Source: CAD feature listing. Evaluate the final solid. Frame: model axes, mm. A direction names the side the tool comes from. Give positions to 0.01 mm unless a question says otherwise; leave off trailing zeros. Write each loop counter-clockwise with the first axis right and the second up, starting at its lowest first coordinate (ties: lowest second). Pieces come first, ordered by that corner, then holes. Notation, with made-up numbers: (-36.75, 55) -> (-18.75, 55) arc R8 ccw to (-18.75, 67) -> close; hole circle Ø4 at (6, -8.5). An arc over 180 degrees is marked (long way). Answer as a JSON object with one key per item and string values. Group by question number.
Item 1: Access query for faces 4 (the face through (81, 8, -26)), 5 (the face through (191, 4, -71.204)). Directions: +Z, -Z, +X, -X, +Y, -Y. A direction counts if a zero-diameter tool reaches every point of the face in a straight line with its end or side. Return the directions, or none.
Item 2: First-contact query: pin 1 Ø3 at (x, z) = (79.79, -50.39) entering from +Y. Flat tip, straight axial feed; report the tip coordinate or a pass-through.
Item 3: Pull-direction query (Z, two-part tool) for faces 1 (the face through (81, 4, 35.296)), 2 (the face through (191, 4, -68.204)), 3 (the face through (81, 4, -84.704)); classes: pulls with the +Z half, pulls with the -Z half, needs draft (parallel to the pull), parting line crosses it, or undercut.
Item 4: Ray query, probe 1 along X at (y, z) = (7.5, -41); probe 2 along Z at (x, y) = (195.5, 0.5); probe 3 along Z at (x, y) = (213.5, 2.25). Return the intervals inside material, ascending. Write a range as from..to.
Item 5: Section query A-A on z = -19. Return the cut outline in (x, y), plus the area to 3 significant figures.
Item 6: Section query B-B on y = 6.75. Give the number of separate pieces and of enclosed holes in the cut face, plus the area to 3 significant figures.
from build123d import *

# Parameters (mm, degrees)
SKETCH1_W           = 300
SKETCH1_H           = 120
BOSS_EXTRUDE1_DEPTH = 8
SKETCH2_R           = 1.636
SKETCH2_R_2         = 1.687
CUT_EXTRUDE1_DEPTH  = 8
CUT_EXTRUDE2_DEPTH  = 8
CUT_EXTRUDE3_DEPTH  = 8
SKETCH2_5_R         = 1.636
CUT_EXTRUDE4_DEPTH  = 8
SKETCH5_R           = 2
CUT_EXTRUDE5_DEPTH  = 8
SKETCH5_3_R         = 2
CUT_EXTRUDE6_DEPTH  = 8
CUT_EXTRUDE7_DEPTH  = 8
SKETCH9_R           = 1.5
CUT_EXTRUDE9_DEPTH  = 10
SKETCH8_R           = 1.5
CUT_EXTRUDE10_DEPTH = 10
SKETCH10_R          = 1.687
SKETCH10_R_2        = 1.636
CUT_EXTRUDE11_DEPTH = 10
SKETCH10_3_R        = 2
CUT_EXTRUDE12_DEPTH = 10
SKETCH10_4_R        = 2
CUT_EXTRUDE13_DEPTH = 10


with BuildPart() as part:
    # Sketch1 → Boss-Extrude1 (new body)
    with BuildSketch(Plane(origin=(0, 0, 0), x_dir=(1, 0, 0), z_dir=(0, 1, 0))):
        with Locations((83.012516048, 24.703699284)):
            Rectangle(SKETCH1_W, SKETCH1_H)
    extrude(amount=BOSS_EXTRUDE1_DEPTH)

    # Sketch2 → Cut-Extrude1 (cut)
    with BuildSketch(Plane(origin=(0, 8, 0), x_dir=(1, 0, 0), z_dir=(0, 1, 0))):
        with Locations((79.785470733, 50.392260228)):
            Circle(SKETCH2_R)
        with Locations((74.502270733, 49.630260228)):
            Circle(SKETCH2_R_2)
        with Locations((81.055470733, 2.132260228)):
            Circle(SKETCH2_R)
        with Locations((155.985470733, 2.132260228)):
            Circle(SKETCH2_R)
    extrude(amount=-CUT_EXTRUDE1_DEPTH, mode=Mode.SUBTRACT)

    # Sketch2<3> → Cut-Extrude2 (cut)
    with BuildSketch(Plane(origin=(0, 8, 0), x_dir=(1, 0, 0), z_dir=(0, 1, 0))):
        with BuildLine():
            Line((-58.487483952, -8.046300716), (-58.487483952, 57.453699284))
            ThreePointArc((-58.487483952, 57.453699284), (-56.987483952, 58.953699284), (-55.487483952, 57.453699284))
            Line((-55.487483952, 57.453699284), (-55.487483952, -8.046300716))
            ThreePointArc((-55.487483952, -8.046300716), (-56.987483952, -9.546300716), (-58.487483952, -8.046300716))
        make_face()
    extrude(amount=-CUT_EXTRUDE2_DEPTH, mode=Mode.SUBTRACT)

    # Sketch2<4> → Cut-Extrude3 (cut)
    with BuildSketch(Plane(origin=(0, 8, 0), x_dir=(1, 0, 0), z_dir=(0, 1, 0))):
        with BuildLine():
            Line((126.512516048, -8.046300716), (126.512516048, 57.453699284))
            ThreePointArc((126.512516048, 57.453699284), (128.012516048, 58.953699284), (129.512516048, 57.453699284))
            Line((129.512516048, 57.453699284), (129.512516048, -8.046300716))
            ThreePointArc((129.512516048, -8.046300716), (128.012516048, -9.546300716), (126.512516048, -8.046300716))
        make_face()
    extrude(amount=-CUT_EXTRUDE3_DEPTH, mode=Mode.SUBTRACT)

    # Sketch2<5> → Cut-Extrude4 (cut)
    with BuildSketch(Plane(origin=(0, 8, 0), x_dir=(1, 0, 0), z_dir=(0, 1, 0))):
        with Locations((162.335470733, 50.392260228)):
            Circle(SKETCH2_5_R)
    extrude(amount=-CUT_EXTRUDE4_DEPTH, mode=Mode.SUBTRACT)

    # Sketch5 → Cut-Extrude5 (cut)
    with BuildSketch(Plane(origin=(0, 8, 0), x_dir=(1, 0, 0), z_dir=(0, 1, 0))):
        with Locations((83.012516048, -20.296300716)):
            Circle(SKETCH5_R)
    extrude(amount=-CUT_EXTRUDE5_DEPTH, mode=Mode.SUBTRACT)

    # Sketch5<3> → Cut-Extrude6 (cut)
    with BuildSketch(Plane(origin=(0, 8, 0), x_dir=(1, 0, 0), z_dir=(0, 1, 0))):
        with Locations((83.012516048, 69.703699284)):
            Circle(SKETCH5_3_R)
    extrude(amount=-CUT_EXTRUDE6_DEPTH, mode=Mode.SUBTRACT)

    # Sketch6 → Cut-Extrude7 (cut)
    with BuildSketch(Plane(origin=(0, 8, 0), x_dir=(1, 0, 0), z_dir=(0, 1, 0))):
        with BuildLine():
            Line((180.768543767, 71.203699284), (201.803443745, 71.203699284))
            ThreePointArc((201.803443745, 71.203699284), (203.303443745, 69.703699284), (201.803443745, 68.203699284))
            Line((201.803443745, 68.203699284), (180.768543767, 68.203699284))
            ThreePointArc((180.768543767, 68.203699284), (179.268543767, 69.703699284), (180.768543767, 71.203699284))
        make_face()
        with BuildLine():
            Line((180.768543767, -18.796300716), (200.303443745, -18.796300716))
            ThreePointArc((200.303443745, -18.796300716), (201.803443745, -20.296300716), (200.303443745, -21.796300716))
            Line((200.303443745, -21.796300716), (180.768543767, -21.796300716))
            ThreePointArc((180.768543767, -21.796300716), (179.268543767, -20.296300716), (180.768543767, -18.796300716))
        make_face()
    extrude(amount=-CUT_EXTRUDE7_DEPTH, mode=Mode.SUBTRACT)

    # Sketch9 → Cut-Extrude9 (cut)
    with BuildSketch(Plane.XZ):
        with Locations((213.012516048, -79.703699284)):
            Circle(SKETCH9_R)
        with Locations((-46.987483952, -79.703699284)):
            Circle(SKETCH9_R)
    extrude(amount=-CUT_EXTRUDE9_DEPTH, mode=Mode.SUBTRACT)

    # Sketch8 → Cut-Extrude10 (cut)
    with BuildSketch(Plane(origin=(0, 8, 0), x_dir=(1, 0, 0), z_dir=(0, 1, 0))):
        with Locations((-46.987483952, -30.296300716)):
            Circle(SKETCH8_R)
        with Locations((213.012516048, -30.296300716)):
            Circle(SKETCH8_R)
    extrude(amount=-CUT_EXTRUDE10_DEPTH, mode=Mode.SUBTRACT)

    # Sketch10 → Cut-Extrude11 (cut)
    with BuildSketch(Plane.XZ):
        with Locations((51.875302079, -49.630260228)):
            Circle(SKETCH10_R)
        with Locations((57.158502079, -50.392260228)):
            Circle(SKETCH10_R_2)
        with Locations((58.428502079, -2.132260228)):
            Circle(SKETCH10_R_2)
        with Locations((139.708502079, -50.392260228)):
            Circle(SKETCH10_R_2)
        with Locations((133.358502079, -2.132260228)):
            Circle(SKETCH10_R_2)
    extrude(amount=-CUT_EXTRUDE11_DEPTH, mode=Mode.SUBTRACT)

    # Sketch10<3> → Cut-Extrude12 (cut)
    with BuildSketch(Plane.XZ):
        with Locations((207.512516048, 22.296300716)):
            Circle(SKETCH10_3_R)
    extrude(amount=-CUT_EXTRUDE12_DEPTH, mode=Mode.SUBTRACT)

    # Sketch10<4> → Cut-Extrude13 (cut)
    with BuildSketch(Plane.XZ):
        with Locations((-41.487483952, 22.296300716)):
            Circle(SKETCH10_4_R)
        with Locations((-41.487483952, -71.703699284)):
            Circle(SKETCH10_4_R)
    extrude(amount=-CUT_EXTRUDE13_DEPTH, mode=Mode.SUBTRACT)


solid = part.part
Worked answers:
{
 "1": {"face 4": "+Z, -Z, +X, -X, +Y", "face 5": "+Y, -Y"},
 "2": {"pin 1": "through"},
 "3": {"face 1": "pulls with the +Z half", "face 2": "undercut", "face 3": "pulls with the -Z half"},
 "4": {"probe 1": "-66.99..-58.49, -55.49..126.51, 129.51..233.01", "probe 2": "-84.7..-71.2, -68.2..18.8, 21.8..35.3", "probe 3": "-84.7..-81.12, -78.29..28.88, 31.71..35.3"},
 "5": {"outline": "(-66.99, 0) -> (-58.49, 0) -> (-58.49, 8) -> (-66.99, 8) -> close; (-55.49, 0) -> (126.51, 0) -> (126.51, 8) -> (-55.49, 8) -> close; (129.51, 0) -> (233.01, 0) -> (233.01, 8) -> (129.51, 8) -> close", "area": "2,350 mm^2"},
 "6": {"separate pieces": "1", "enclosed holes": "23", "area": "35,300 mm^2"}
}
